Geometry: final body of the model. Coordinates: model frame, mm. Face numbers are marked on the shaded views. A direction names the side the tool comes from. Give positions to 0.01 mm unless a question says otherwise; leave off trailing zeros. Write each loop counter-clockwise with the first axis right and the second up, starting at its lowest first coordinate (ties: lowest second). Pieces come first, ordered by that corner, then holes. Notation, with made-up numbers: (-7, 68.5) -> (2, 68.5) arc R20 cw to (2, 107.5) -> close; hole circle Ø8 at (-38.75, 34.25). An arc over 180 degrees is marked (long way). Answer as a JSON object with one key per item and string values. Group by question number.
(1) Section query D-D on z = -10. Output: boundary loops of the cut face in (x, y), plus the area to 3 significant figures.
(2) Material intervals for probe 1 along Z at (x, y) = (10.5, 35); probe 2 along X at (y, z) = (-39, -2); probe 3 along Y at (x, z) = (16, 0), sorted ascending.
(3) Section query C-C on y = 11. Output: boundary loops of the cut face in (x, z).
(4) Section query B-B on x = -0.5. Output: boundary loops of the cut face in (y, z).
(5) Set-up query: the marked faces 4 and 5. Return all of +Z, -Z, +X, -X, +Y, -Y with unobstructed straight access to the full face (end or side cutting, diameter ignored); none if empty.
(6) Draft query along Y for the marked faces 1, 2 and 3. Return one class per face: +Y half, -Y half, draft (parallel to the pull), parting line (faces both ways), or undercut.
(7) Section query A-A on y = -23.5. Output: boundary loops of the cut face in (x, z).
(8) Contact query for flat-ended pins moving along their axis: pin 1 Ø10 at (x, y) = (-10, -29.5) entering from -Z; pin 2 Ø2 at (x, z) = (15.5, 0.5) entering from +Y; pin 3 Ø2.5 at (x, z) = (1.5, -1.5) entering from -Y; pin 4 Ø10.5 at (y, z) = (-59.5, -0.5) entering from -X. Output: stop coordinate, or through.
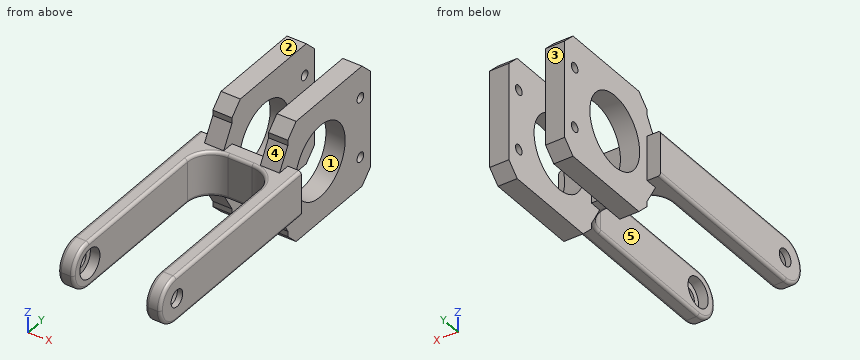
from build123d import *

# Parameters (mm, degrees)
SKETCH_1_W          = 34
SKETCH_1_H          = 15
EXTRUDE_1_DEPTH     = 68
SKETCH_3_W          = 24
SKETCH_3_H          = 63
CUT_EXTRUDE_1_DEPTH = 72.67984375
FILLET_1_R          = 8
FILLET_3_R          = 7.5
FILLET_2_R          = 1
SKETCH_4_R          = 2.8
CUT_EXTRUDE_2_DEPTH = 77.395353351
SKETCH_6_R          = 4.85
CUT_EXTRUDE_4_DEPTH = 3.2
SKETCH_7_W          = 40.44939287
SKETCH_7_H          = 39.770190269
SKETCH_7_R          = 12
SKETCH_7_R_2        = 1.6
EXTRUDE_2_DEPTH     = 12.5
SKETCH_8_W          = 12.191161996
SKETCH_8_H          = 39.770190269
CUT_EXTRUDE_5_DEPTH = 81.926839783
CHAMFER_1_SIZE      = 4
CHAMFER_1_SIZE_2    = 6.92820323
CHAMFER_2_SIZE      = 4


# Some blends are built 0.0001 mm under size
with BuildPart() as part:
    # 草图1 → 凸台-拉伸1 (new body)
    with BuildSketch(Plane(origin=(0, 0, 0), x_dir=(1, 0, 0), z_dir=(0, 1, 0))):
        Rectangle(SKETCH_1_W, SKETCH_1_H)
    extrude(amount=-EXTRUDE_1_DEPTH)

    # 草图3 → 切除-拉伸1 (cut, through all)
    with BuildSketch(Plane.XY.offset(7.5)):
        with Locations((0, -36.5)):
            Rectangle(SKETCH_3_W, SKETCH_3_H)
    extrude(amount=-CUT_EXTRUDE_1_DEPTH, mode=Mode.SUBTRACT)

    # 圆角1
    fillet_1_edges = [part.edges().sort_by_distance(p)[0] for p in [
        (-12, -5, 0),
        (12, -5, 0),
    ]]
    fillet(fillet_1_edges, radius=FILLET_1_R)

    # 圆角3
    fillet_3_edges = [part.edges().sort_by_distance(p)[0] for p in [
        (14.5, -68, -7.5),
        (14.5, -68, 7.5),
        (-14.5, -68, -7.5),
        (-14.5, -68, 7.5),
    ]]
    fillet(fillet_3_edges, radius=FILLET_3_R - 0.0001)  # a hair under: the kernel refuses the full size

    # 圆角2
    fillet_2_edges = [part.edges().sort_by_distance(p)[0] for p in [
        (0, -5, 7.5),
        (0, -5, -7.5),
        (-12, -36.75005, 7.5),
        (-12, -36.75005, -7.5),
        (9.656854249, -7.343145751, 7.5),
        (9.656854249, -7.343145751, -7.5),
        (-9.656854249, -7.343145751, 7.5),
        (-9.656854249, -7.343145751, -7.5),
        (-17, -30.25005, -7.5),
        (17, -30.25005, -7.5),
        (12, -36.75005, -7.5),
        (12, -36.75005, 7.5),
        (12, -65.803330148, 5.303330148),
        (12, -65.803330148, -5.303330148),
        (17, -30.25005, 7.5),
        (17, -65.803330148, 5.303330148),
        (17, -65.803330148, -5.303330148),
        (-17, -30.25005, 7.5),
        (-17, -65.803330148, 5.303330148),
        (-17, -65.803330148, -5.303330148),
        (-12, -65.803330148, 5.303330148),
        (-12, -65.803330148, -5.303330148),
    ]]
    fillet(fillet_2_edges, radius=FILLET_2_R)

    # 草图4 → 切除-拉伸2 (cut, through all)
    with BuildSketch(Plane(origin=(17, 0, 0), x_dir=(0, 0, -1), z_dir=(1, 0, 0))):
        with Locations((0, -60)):
            Circle(SKETCH_4_R)
    extrude(amount=-CUT_EXTRUDE_2_DEPTH, mode=Mode.SUBTRACT)

    # 草图6 → 切除-拉伸4 (cut)
    with BuildSketch(Plane(origin=(12, 0, 0), x_dir=(0, 0, -1), z_dir=(1, 0, 0))):
        with Locations((0, -60)):
            Circle(SKETCH_6_R)
    cut_extrude_4 = extrude(amount=CUT_EXTRUDE_4_DEPTH, mode=Mode.SUBTRACT)

    # 镜向1: 切除-拉伸4 across plane
    add(cut_extrude_4.mirror(Plane(origin=(0, 0, 0), x_dir=(0, 0, 1), z_dir=(1, 0, 0))), mode=Mode.SUBTRACT)

    # 草图7 → 凸台-拉伸2 (add, symmetric)
    with BuildSketch(Plane(origin=(0, 0, 0), x_dir=(0, 0, -1), z_dir=(1, 0, 0))):
        with Locations((0, 19.885095135)):
            Rectangle(SKETCH_7_W, SKETCH_7_H)
        with Locations((0, 15.650854712)):
            Circle(SKETCH_7_R, mode=Mode.SUBTRACT)
        with Locations((-10, 35)):
            Circle(SKETCH_7_R_2, mode=Mode.SUBTRACT)
        with Locations((10, 35)):
            Circle(SKETCH_7_R_2, mode=Mode.SUBTRACT)
    extrude(amount=EXTRUDE_2_DEPTH, both=True)

    # 草图8 → 切除-拉伸5 (cut, through all)
    with BuildSketch(Plane.XY.offset(20.224696435)):
        with Locations((0, 19.885095135)):
            Rectangle(SKETCH_8_W, SKETCH_8_H)
    extrude(amount=-CUT_EXTRUDE_5_DEPTH, mode=Mode.SUBTRACT)

    # 倒角1
    # the kernel refuses this chamfer: 6.92820323, 4 mm, written as the material it adds along each edge
    with BuildSketch(Plane(origin=(-12.5, 0, 7.5), x_dir=(0, -0.9983227437537926, -0.057893862402671484), z_dir=(1, 0, 0)), Plane(origin=(6.095580998, 0, 7.5), x_dir=(0, -0.9983227437537926, -0.057893862402671484), z_dir=(1, 0, 0)), Plane(origin=(12.5, 0, -7.5), x_dir=(0, -0.9983227437537926, 0.057893862402671484), z_dir=(-1, 0, 0)), Plane(origin=(-6.095580998, 0, -7.5), x_dir=(0, -0.9983227437537926, 0.057893862402671484), z_dir=(-1, 0, 0))) as chamfer_1_piece_1:
        Polygon((CHAMFER_1_SIZE * 0.998322743754, -CHAMFER_1_SIZE * 0.0578938624027), (-CHAMFER_1_SIZE_2 * 0.057893862405, -CHAMFER_1_SIZE_2 * 0.998322743793), (0, 0), align=None)
    extrude(amount=6.404419002)
    with BuildSketch(Plane(origin=(-30.423855882, 0, 7.5), x_dir=(0, -0.9983227437537926, -0.057893862402671484), z_dir=(1, 0, 0))) as chamfer_1_piece_2_section:
        Polygon((CHAMFER_1_SIZE * 0.998322743754, -CHAMFER_1_SIZE * 0.0578938624027), (-CHAMFER_1_SIZE_2 * 0.057893862405, -CHAMFER_1_SIZE_2 * 0.998322743793), (0, 0), align=None)
    chamfer_1_piece_2 = extrude(amount=42.252130767, mode=Mode.PRIVATE)
    chamfer_1_piece_2 = split(chamfer_1_piece_2, bisect_by=Plane(origin=(6.095580998, -1.333333333, 9.809401077), z_dir=(1, 0, 0)), keep=Keep.TOP, mode=Mode.PRIVATE)
    add(chamfer_1_piece_2)
    with BuildSketch(Plane(origin=(-11.828274885, 0, 7.5), x_dir=(0, -0.9983227437537926, -0.057893862402671484), z_dir=(1, 0, 0))) as chamfer_1_piece_3_section:
        Polygon((CHAMFER_1_SIZE * 0.998322743754, -CHAMFER_1_SIZE * 0.0578938624027), (-CHAMFER_1_SIZE_2 * 0.057893862405, -CHAMFER_1_SIZE_2 * 0.998322743793), (0, 0), align=None)
    chamfer_1_piece_3 = extrude(amount=42.252130767, mode=Mode.PRIVATE)
    chamfer_1_piece_3 = split(chamfer_1_piece_3, bisect_by=Plane(origin=(-6.095580998, -1.333333333, 9.809401077), z_dir=(-1, 0, 0)), keep=Keep.TOP, mode=Mode.PRIVATE)
    add(chamfer_1_piece_3)
    with BuildSketch(Plane(origin=(30.423855882, 0, -7.5), x_dir=(0, -0.9983227437537926, 0.057893862402671484), z_dir=(-1, 0, 0))) as chamfer_1_piece_4_section:
        Polygon((CHAMFER_1_SIZE * 0.998322743754, -CHAMFER_1_SIZE * 0.0578938624027), (-CHAMFER_1_SIZE_2 * 0.057893862405, -CHAMFER_1_SIZE_2 * 0.998322743793), (0, 0), align=None)
    chamfer_1_piece_4 = extrude(amount=42.252130767, mode=Mode.PRIVATE)
    chamfer_1_piece_4 = split(chamfer_1_piece_4, bisect_by=Plane(origin=(-6.095580998, -1.333333333, -9.809401077), z_dir=(-1, 0, 0)), keep=Keep.TOP, mode=Mode.PRIVATE)
    add(chamfer_1_piece_4)
    with BuildSketch(Plane(origin=(11.828274885, 0, -7.5), x_dir=(0, -0.9983227437537926, 0.057893862402671484), z_dir=(-1, 0, 0))) as chamfer_1_piece_5_section:
        Polygon((CHAMFER_1_SIZE * 0.998322743754, -CHAMFER_1_SIZE * 0.0578938624027), (-CHAMFER_1_SIZE_2 * 0.057893862405, -CHAMFER_1_SIZE_2 * 0.998322743793), (0, 0), align=None)
    chamfer_1_piece_5 = extrude(amount=42.252130767, mode=Mode.PRIVATE)
    chamfer_1_piece_5 = split(chamfer_1_piece_5, bisect_by=Plane(origin=(6.095580998, -1.333333333, -9.809401077), z_dir=(1, 0, 0)), keep=Keep.TOP, mode=Mode.PRIVATE)
    add(chamfer_1_piece_5)

    # 倒角2
    chamfer_2_edges = [part.edges().sort_by_distance(p)[0] for p in [
        (9.297790499, 0, 20.224696435),
        (9.297790499, 39.770190269, 20.224696435),
        (9.297790499, 0, -20.224696435),
        (9.297790499, 39.770190269, -20.224696435),
        (-9.297790499, 39.770190269, 20.224696435),
        (-9.297790499, 39.770190269, -20.224696435),
        (-9.297790499, 0, -20.224696435),
        (-9.297790499, 0, 20.224696435),
    ]]
    chamfer(chamfer_2_edges, length=CHAMFER_2_SIZE)


solid = part.part
Answer list:
{
 "1": {"outline": "(-12.5, -2.56) -> (-6.1, -2.56) -> (-6.1, 9.02) -> (-12.5, 9.02) -> close; (-12.5, 22.28) -> (-6.1, 22.28) -> (-6.1, 33.4) -> (-12.5, 33.4) -> close; (-12.5, 36.6) -> (-6.1, 36.6) -> (-6.1, 39.77) -> (-12.5, 39.77) -> close; (6.1, -2.56) -> (12.5, -2.56) -> (12.5, 9.02) -> (6.1, 9.02) -> close; (6.1, 22.28) -> (12.5, 22.28) -> (12.5, 33.4) -> (6.1, 33.4) -> close; (6.1, 36.6) -> (12.5, 36.6) -> (12.5, 39.77) -> (6.1, 39.77) -> close", "area": "331 mm2"},
 "2": {"probe 1": "-20.22 to -11.6, -8.4 to 8.4, 11.6 to 20.22", "probe 2": "-17 to -12, 12 to 17", "probe 3": "-68 to -62.8, -57.2 to 0"},
 "3": {"outline": "(-12.5, -20.22) -> (-6.1, -20.22) -> (-6.1, -11.06) -> (-12.5, -11.06) -> close; (-12.5, 11.06) -> (-6.1, 11.06) -> (-6.1, 20.22) -> (-12.5, 20.22) -> close; (6.1, -20.22) -> (12.5, -20.22) -> (12.5, -11.06) -> (6.1, -11.06) -> close; (6.1, 11.06) -> (12.5, 11.06) -> (12.5, 20.22) -> (6.1, 20.22) -> close"},
 "4": {"outline": "(-5, -6.5) arc R1 ccw to (-4, -7.5) -> (0, -7.5) -> (0, 7.5) -> (-4, 7.5) arc R1 ccw to (-5, 6.5) -> close"},
 "5": {"face 4": "+Z, +X, -X, -Y", "face 5": "+Z, -Z, -Y"},
 "6": {"face 1": "undercut", "face 2": "draft", "face 3": "+Y half"},
 "7": {"outline": "(-17, -6.5) arc R1 ccw to (-16, -7.5) -> (-13, -7.5) arc R1 ccw to (-12, -6.5) -> (-12, 6.5) arc R1 ccw to (-13, 7.5) -> (-16, 7.5) arc R1 ccw to (-17, 6.5) -> close; (12, -6.5) arc R1 ccw to (13, -7.5) -> (16, -7.5) arc R1 ccw to (17, -6.5) -> (17, 6.5) arc R1 ccw to (16, 7.5) -> (13, 7.5) arc R1 ccw to (12, 6.5) -> close"},
 "8": {"pin 1": "z = -7.5", "pin 2": "y = 0", "pin 3": "y = -5", "pin 4": "x = -17"}
}
